For this review, take the finished solid that the model builds, in its own axes (mm). Face numbers are marked on the shaded views. A direction names the side the tool comes from. Give positions to 0.01 mm unless a question says otherwise; leave off trailing zeros. Write each loop counter-clockwise with the first axis right and the second up, starting at its lowest first coordinate (ties: lowest second). Pieces come first, ordered by that corner, then holes. Notation, with made-up numbers: (77, 44.25) -> (102, 44.25) arc R14 ccw to (102, 70.25) -> close; hole circle Ø1 at (12.5, 54). An arc over 180 degrees is marked (long way). Answer as CSV lines item,"result".
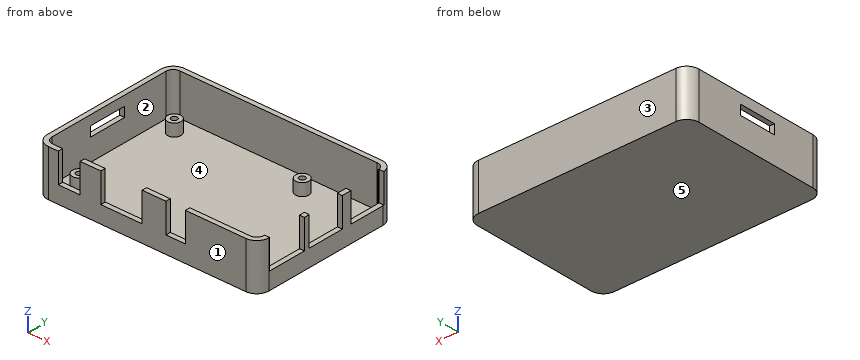
```python
from build123d import *

# Parameters (mm, degrees)
F1_DEPTH = 2
F2_DEPTH = 19
F3_R     = 2.75
F3_R_2   = 1.25
F4_DEPTH = 5
F5_W     = 9
F5_H     = 2
F5_W_2   = 2
F5_H_2   = 15.1
F5_W_3   = 17
F5_W_4   = 8
F5_H_3   = 15.9
F6_DEPTH = 12
F7_W     = 15.6
F7_H     = 4
F8_DEPTH = 25


with BuildPart() as f1:
    # F0 (on Top) → F1 (new body)
    with BuildSketch(Plane.XY):
        with BuildLine():
            ThreePointArc((0, 5), (1.4644660941, 1.4644660941), (5, 0))
            Line((5, 0), (86, 0))
            ThreePointArc((86, 0), (89.5355339059, 1.4644660941), (91, 5))
            Line((91, 5), (91, 57))
            ThreePointArc((91, 57), (89.5355339059, 60.5355339059), (86, 62))
            Line((86, 62), (5, 62))
            ThreePointArc((5, 62), (1.4644660941, 60.5355339059), (0, 57))
            Line((0, 57), (0, 5))
        make_face()
        with BuildLine():
            ThreePointArc((2, 57), (2.8786796564, 59.1213203436), (5, 60))
            Line((5, 60), (86, 60))
            ThreePointArc((86, 60), (88.1213203436, 59.1213203436), (89, 57))
            Line((89, 57), (89, 5))
            ThreePointArc((89, 5), (88.1213203436, 2.8786796564), (86, 2))
            Line((86, 2), (5, 2))
            ThreePointArc((5, 2), (2.8786796564, 2.8786796564), (2, 5))
            Line((2, 5), (2, 57))
        make_face(mode=Mode.SUBTRACT)
        with BuildLine():
            Line((86, 60), (5, 60))
            ThreePointArc((5, 60), (2.8786796564, 59.1213203436), (2, 57))
            Line((2, 57), (2, 5))
            ThreePointArc((2, 5), (2.8786796564, 2.8786796564), (5, 2))
            Line((5, 2), (86, 2))
            ThreePointArc((86, 2), (88.1213203436, 2.8786796564), (89, 5))
            Line((89, 5), (89, 57))
            ThreePointArc((89, 57), (88.1213203436, 59.1213203436), (86, 60))
        make_face()
    extrude(amount=F1_DEPTH)

    # F0 (on Top) → F2 (join)
    with BuildSketch(Plane.XY):
        with BuildLine():
            ThreePointArc((0, 5), (1.4644660941, 1.4644660941), (5, 0))
            Line((5, 0), (86, 0))
            ThreePointArc((86, 0), (89.5355339059, 1.4644660941), (91, 5))
            Line((91, 5), (91, 57))
            ThreePointArc((91, 57), (89.5355339059, 60.5355339059), (86, 62))
            Line((86, 62), (5, 62))
            ThreePointArc((5, 62), (1.4644660941, 60.5355339059), (0, 57))
            Line((0, 57), (0, 5))
        make_face()
        with BuildLine():
            ThreePointArc((2, 57), (2.8786796564, 59.1213203436), (5, 60))
            Line((5, 60), (86, 60))
            ThreePointArc((86, 60), (88.1213203436, 59.1213203436), (89, 57))
            Line((89, 57), (89, 5))
            ThreePointArc((89, 5), (88.1213203436, 2.8786796564), (86, 2))
            Line((86, 2), (5, 2))
            ThreePointArc((5, 2), (2.8786796564, 2.8786796564), (2, 5))
            Line((2, 5), (2, 57))
        make_face(mode=Mode.SUBTRACT)
    extrude(amount=F2_DEPTH)

    # F3 (on face) → F4 (join)
    with BuildSketch(Plane.XY.offset(2)):
        with Locations((9.25, 52.75)):
            Circle(F3_R)
        with Locations((9.25, 52.75)):
            Circle(F3_R_2, mode=Mode.SUBTRACT)
        with Locations((9.25, 9.25)):
            Circle(F3_R)
        with Locations((9.25, 9.25)):
            Circle(F3_R_2, mode=Mode.SUBTRACT)
        with Locations((61.75, 9.25)):
            Circle(F3_R)
        with Locations((61.75, 9.25)):
            Circle(F3_R_2, mode=Mode.SUBTRACT)
        with Locations((61.75, 52.75)):
            Circle(F3_R)
        with Locations((61.75, 52.75)):
            Circle(F3_R_2, mode=Mode.SUBTRACT)
    extrude(amount=F4_DEPTH)

    # F5 (on face) → F6 (cut)
    with BuildSketch(Plane.XY.offset(19)):
        with Locations((13.55, 1)):
            Rectangle(F5_W, F5_H)
        with Locations((90, 49.95)):
            Rectangle(F5_W_2, F5_H_2)
        with Locations((35, 1)):
            Rectangle(F5_W_3, F5_H)
        with Locations((57.25, 1)):
            Rectangle(F5_W_4, F5_H)
        with Locations((90, 13.25)):
            Rectangle(F5_W_2, F5_H_3)
        with Locations((90, 30.95)):
            Rectangle(F5_W_2, F5_H_2)
    extrude(amount=-F6_DEPTH, mode=Mode.SUBTRACT)

    # F7 (on face) → F8 (cut)
    with BuildSketch(Plane(origin=(0, 0, 0), x_dir=(0, -1, 0), z_dir=(-1, 0, 0))):
        with Locations((-30.3, 13)):
            Rectangle(F7_W, F7_H)
    extrude(amount=-F8_DEPTH, mode=Mode.SUBTRACT)


solid = f1.part
```
Q1. Add section C-C (z = 8). State how many separate pieces and enclosed holes the cut face has, plus the area to 3 significant figures.
Answer block:
separate pieces,"6"
enclosed holes,"0"
area,"422 mm2"
Q2. Clearance check with flat-ended pins moving along their axes: pin 1 (3 mm diameter, centred on x = 61.5, y = 9, fed in from +Z); pin 2 (1.6 mm diameter, centred on y = 0.5, z = 15, fed in from +X); pin 3 (6 mm diameter, centred on x = 79.5, y = 21.5, fed in from +Z). State where each tip first meets the part, or that it passes through.
Answer block:
pin 1,"stops at z = 7"
pin 2,"stops at x = 89.36"
pin 3,"stops at z = 2"
Q3. Draft analysis for pull direction Y (two halves, no side actions). For the marked faces 3, 4 and 5, state which applies: released by +Y, released by -Y, zero draft, split by the parting line, or undercut.
Answer block:
face 3,"released by +Y"
face 4,"undercut"
face 5,"zero draft"
Q4. For the marked faces 1 and 2, list the 3-axis set-ups (+Z, -Z, +X, -X, +Y, -Y) from which the entire face can be reached by the end or side of a thin tool; tool diameter is ignored.
Answer block:
face 1,"+Z, -Z, +X, -X, -Y"
face 2,"+Z"
Q5. Add section A-A (y = 33). Write out the cut boundary in (x, z).
Answer block:
outline,"(0, 0) -> (91, 0) -> (91, 7) -> (89, 7) -> (89, 2) -> (2, 2) -> (2, 11) -> (0, 11) -> close; (0, 15) -> (2, 15) -> (2, 19) -> (0, 19) -> close"
Q6. Add section B-B (y = 9.25). Write out the cut boundary in (x, z).
Answer block:
outline,"(0, 0) -> (91, 0) -> (91, 7) -> (89, 7) -> (89, 2) -> (64.5, 2) -> (64.5, 7) -> (63, 7) -> (63, 2) -> (60.5, 2) -> (60.5, 7) -> (59, 7) -> (59, 2) -> (12, 2) -> (12, 7) -> (10.5, 7) -> (10.5, 2) -> (8, 2) -> (8, 7) -> (6.5, 7) -> (6.5, 2) -> (2, 2) -> (2, 19) -> (0, 19) -> close"
Q7. To check wall thickness, follow probe 1 along Y at (x, z) = (61.75, 3.5); probe 2 along Y at (x, z) = (45, 13); probe 3 along Y at (x, z) = (60, 2.75). State the ranges of each line that lie inside material, in increasing order. Write a range as [from, to].
Answer block:
probe 1,"y = [0, 2], [6.5, 8], [10.5, 12], [50, 51.5], [54, 55.5], [60, 62]"
probe 2,"y = [0, 2], [60, 62]"
probe 3,"y = [0, 2], [7.13, 11.37], [50.63, 54.87], [60, 62]"
Q8. Add section D-D (x = 70). Write out the cut boundary in (y, z).
Answer block:
outline,"(0, 0) -> (62, 0) -> (62, 19) -> (60, 19) -> (60, 2) -> (2, 2) -> (2, 19) -> (0, 19) -> close"
